Answer from the drawing. Dimensions are ordinates in mm from the lowest x, y and z of the part. A direction names the side the tool comes from. Give positions to 0.01 mm unless a question says otherwise; leave off trailing zeros. Order: outer loops, then holes, each group sorted by start corner. A loop starts at its lowest first (then second) coordinate and runs counter-clockwise, first axis right, second up. Notation, with made-up numbers: (57.5, -31) - (112.5, -31) arc R17 ccw to (112.5, 2) - close; hole circle Ø11 at (-26.75, 37). An arc over 180 degrees is marked (long way). Answer in a Markdown table with one row per item.
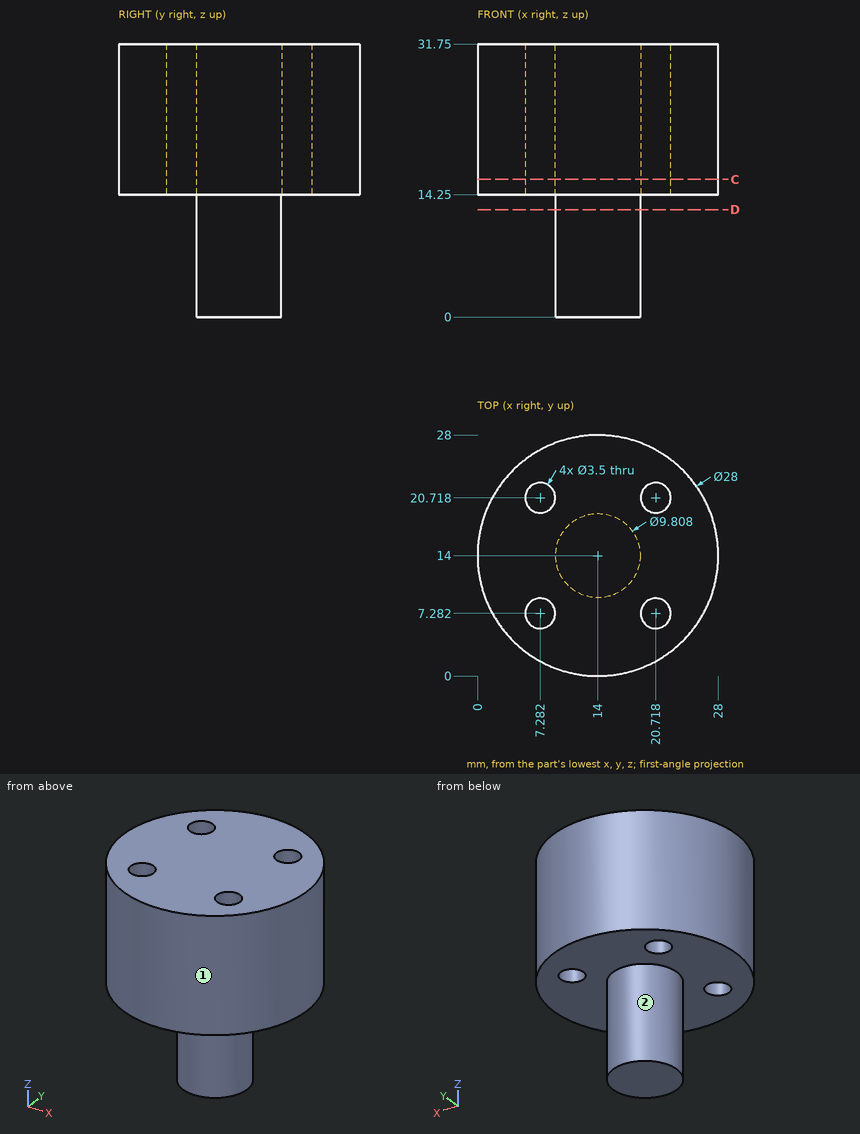
Item 1: Each of these flat-tipped pins is pushed along its axis until it touches: P1, Ø2, axis at y = 18.5, z = 18, coming from the +X side (1 decimal); P2, Ø4, axis at x = 13.5, z = 24, coming from the -Y side; P3, Ø3, axis at x = 20.72, y = 7.28, coming from the -Z side; P4, Ø10, axis at y = 19.5, z = 17.5, coming from the -X side. Where does it stop, or does it pass through?
Answer block:
| item | result |
|---|---|
| P1 | x = 27.6 |
| P2 | y = 0 |
| P3 | through |
| P4 | x = 0.01 |
Item 2: Which of the six approach directions +Z, -Z, +X, -X, +Y, -Y give full straight-line access (tool end or side, diameter ignored) to the marked faces 1 and 2?
Answer block:
| item | result |
|---|---|
| face 1 | +Z, -Z |
| face 2 | -Z |
Item 3: Find section C-C on z = 16. Write down the section's boundary in (x, y), then the cut area to 3 significant figures.
Answer block:
| item | result |
|---|---|
| outline | circle Ø28 at (14, 14); hole circle Ø3.5 at (7.28, 7.28); hole circle Ø3.5 at (7.28, 20.72); hole circle Ø3.5 at (20.72, 7.28); hole circle Ø3.5 at (20.72, 20.72) |
| area | 577 mm² |
Item 4: Consider line 1 (X direction, y = 6.5, z = 29.5) (1 decimal); line 2 (Z direction, x = 13.5, y = 24); line 3 (Y direction, x = 20.5, z = 16) (1 decimal). Determine where each line is inside the solid, lowest interval first.
Answer block:
| item | result |
|---|---|
| line 1 | 2.2 to 5.7, 8.8 to 19.2, 22.3 to 25.8 |
| line 2 | 14.25 to 31.75 |
| line 3 | 1.6 to 5.5, 9 to 19, 22.5 to 26.4 |
Item 5: Find section D-D on z = 12.5. Write down the section's boundary in (x, y) (1 decimal).
Answer block:
| item | result |
|---|---|
| outline | circle Ø9.8 at (14, 14) |
